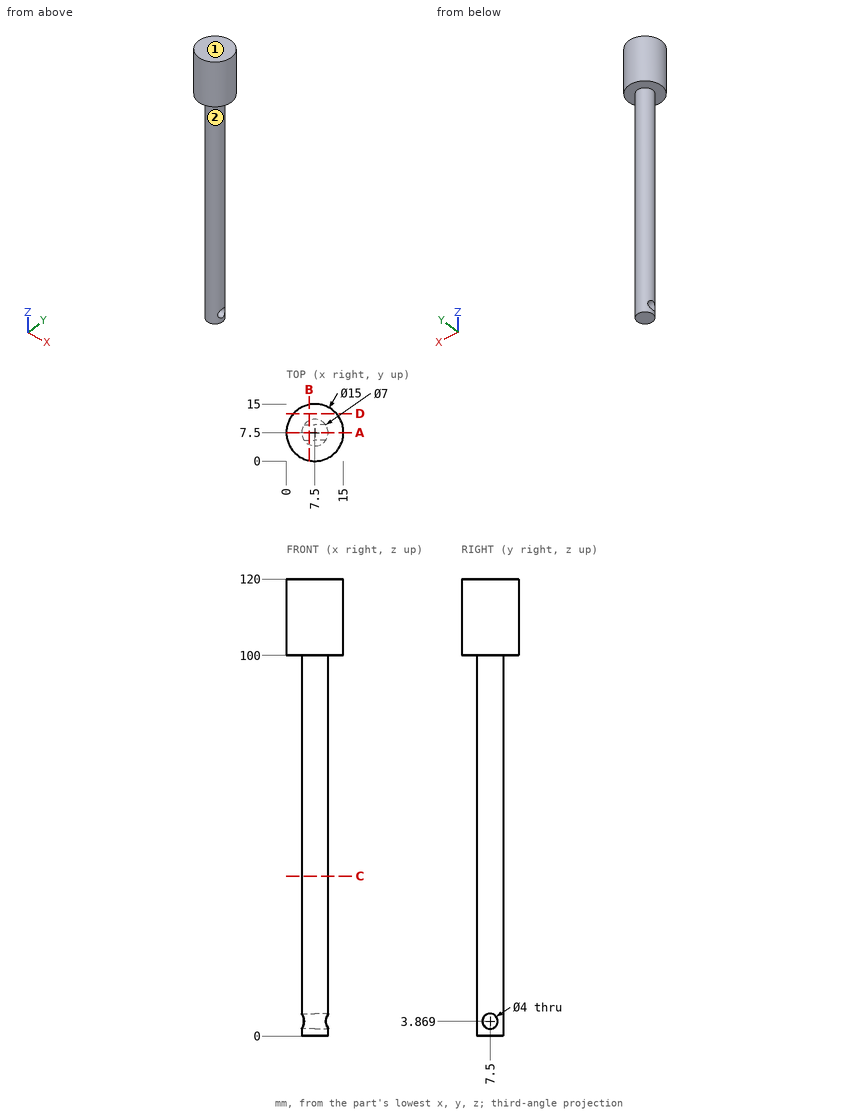
Study the drawing (mm; zero at the part's minimum x, y, z) and answer. A direction names the side the tool comes from. Give positions to 0.01 mm unless a question says otherwise; leave off trailing zeros. Order: outer loops, then holes, each group sorted by start corner. A loop starts at its lowest first (then second) coordinate and runs counter-clockwise, first axis right, second up. Notation, with made-up numbers: (57, 72) - (88, 72) arc R21 ccw to (88, 107) - close; hole circle Ø8 at (-16.75, -15). An arc over 180 degrees is marked (long way). Answer in a Markdown table with one row per item. Add a question column.
Q1. The part is cut by section D-D (y = 12.5). Determine the outline of the cut face in (x, z).
Q2. Find the intervals of material crossed by line 1 along Z through (x, y) = (5.7, 7.5); line 2 along Z through (x, y) = (1.5, 9.75); line 3 along X through (y, z) = (7.75, 43), in increasing order. Write a range as [from, to].
Q3. Given P1, Ø4, axis at x = 6, z = 55.5, coming from the +Y side; P2, Ø3, axis at y = 5, z = 93, coming from the -X side; P3, Ø6, axis at y = 5, z = 68, coming from the -X side, each flat-ended and moving along its own axis, determine where each tip first touches the part or whether it passes through.
Q4. The part is cut by section A-A (y = 7.5). Determine the outline of the cut face in (x, z).
Q5. The part is cut by section B-B (x = 6). Determine the outline of the cut face in (y, z).
Q6. Which of the six approach directions +Z, -Z, +X, -X, +Y, -Y give full straight-line access (tool end or side, diameter ignored) to the marked faces 1 and 2?
Q7. The part is cut by section C-C (z = 42). Determine the outline of the cut face in (x, y).
Determined:
| question | item | result |
|---|---|---|
| 1 | outline | (1.91, 100) - (13.09, 100) - (13.09, 120) - (1.91, 120) - close |
| 2 | line 1 | z = [0, 1.87], [5.87, 120] |
| 2 | line 2 | z = [100, 120] |
| 2 | line 3 | x = [4.01, 10.99] |
| 3 | P1 | stops at y = 11 |
| 3 | P2 | stops at x = 4.15 |
| 3 | P3 | stops at x = 4 |
| 4 | outline | (0, 100) - (4, 100) - (4, 5.87) - (11, 5.87) - (11, 100) - (15, 100) - (15, 120) - (0, 120) - close; (4, 0) - (11, 0) - (11, 1.87) - (4, 1.87) - close |
| 5 | outline | (0.15, 100) - (4.34, 100) - (4.34, 0) - (10.66, 0) - (10.66, 100) - (14.85, 100) - (14.85, 120) - (0.15, 120) - close; hole circle Ø4 at (7.5, 3.87) |
| 6 | face 1 | +Z, +X, -X, +Y, -Y |
| 6 | face 2 | -Z |
| 7 | outline | circle Ø7 at (7.5, 7.5) |
